Could you check a few things on this drawing? It's one solid part, dimensions in mm from its lowest x, y, z. A direction names the side the tool comes from. Round coordinates to 2 decimals unless told otherwise and drop trailing zeros. Loops run counter-clockwise (first coordinate to the right, second up) from the corner with the lowest first, then second, coordinate; pieces in that order, holes last. Notation, with made-up numbers: (47.5, 34) -> (82.5, 34) arc R27 cw to (82.5, 62) -> close; hole circle Ø5 at (63, 83). An arc over 180 degrees is marked (long way). Use one line per item in the form item = value. Start each with the question number.
Item 1: If we section it at D-D (x = 22): Write out the boundary of the cut face in (y, z), then the cut area to 3 significant figures.
Item 2: If we section it at A-A (x = 4): Write out the boundary of the cut face in (y, z).
Item 3: If we section it at B-B (z = 6.75): Write out the boundary of the cut face in (x, y), then the cut area to 3 significant figures.
Item 4: If I drill on L1, parallel to X at y = 6.75, z = 8; L2, parallel to Y at x = 4, z = 1.3; L3, parallel to Y at x = 30, z = 1.3, over which ranges is the centre line in solid material (lowest first)? Write a range as [from, to].
Item 5: For the marked faces 1, 2, 3, 4 and 5, which set-ups out of +Z, -Z, +X, -X, +Y, -Y let a thin tool reach every point of the face, with its end or its side?
Item 6: Thinking about a two-plate mould opening in X: for the marked faces 6, 7, 8 and 9, which applies, released by +X, released by -X, zero draft, split by the parting line, or undercut?
Item 7: If we section it at C-C (y = 17): Write out the boundary of the cut face in (x, z).
Item 8: I'm going to push flat-ended pins straight in: pin 1 Ø4.5 at (y, z) = (5, 6.5) entering from +X; pin 2 Ø1.2 at (x, y) = (15.5, 6) entering from +Z; pin 3 Ø3 at (x, z) = (12.5, 5.5) entering from -Y; pin 4 Ø5 at (y, z) = (11, 9) entering from -X. Where does each tip first touch, or does it pass through?
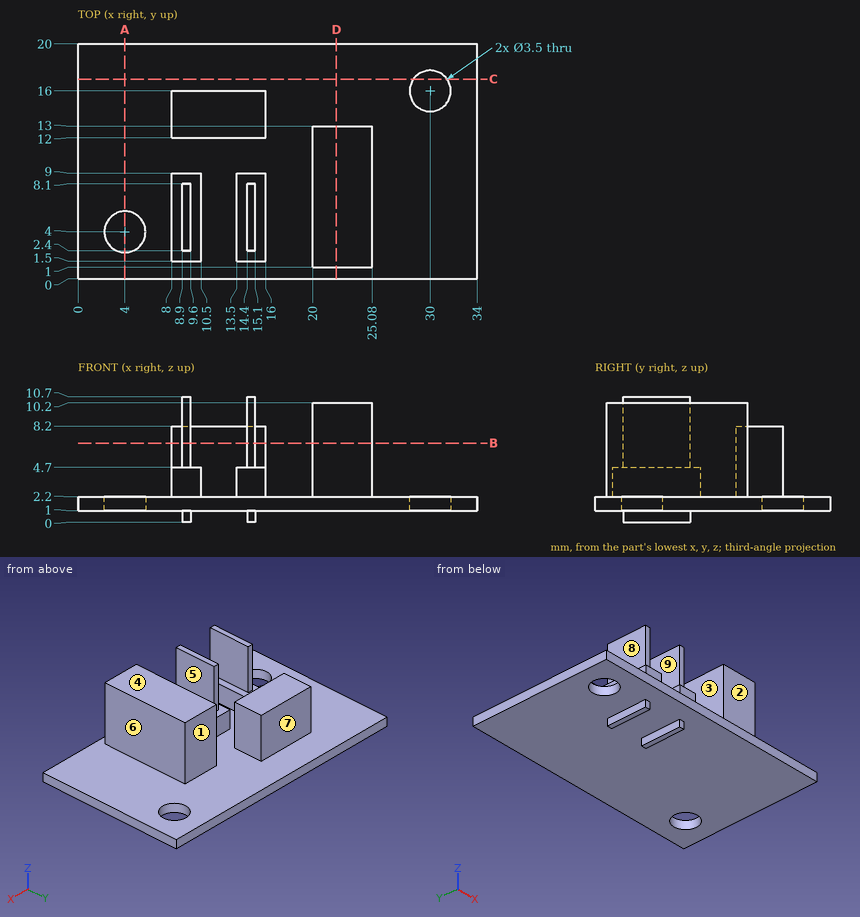
Values found:
q1.outline = (0, 1) -> (20, 1) -> (20, 2.2) -> (13, 2.2) -> (13, 10.2) -> (1, 10.2) -> (1, 2.2) -> (0, 2.2) -> close
q1.area = 120 mm2
q2.outline = (0, 1) -> (2.25, 1) -> (2.25, 2.2) -> (0, 2.2) -> close; (5.75, 1) -> (20, 1) -> (20, 2.2) -> (5.75, 2.2) -> close
q3.outline = (8, 12) -> (16, 12) -> (16, 16) -> (8, 16) -> close; (8.9, 2.4) -> (9.6, 2.4) -> (9.6, 8.1) -> (8.9, 8.1) -> close; (14.4, 2.4) -> (15.1, 2.4) -> (15.1, 8.1) -> (14.4, 8.1) -> close; (20, 1) -> (25.08, 1) -> (25.08, 13) -> (20, 13) -> close
q3.area = 101 mm2
q4.L1 = [8.9, 9.6], [14.4, 15.1], [20, 25.08]
q4.L2 = [0, 2.25], [5.75, 20]
q4.L3 = [0, 14.25], [17.75, 20]
q5.face_1 = +Z, +X, +Y
q5.face_2 = +Z, +X, -X, -Y
q5.face_3 = +Z, +Y, -Y
q5.face_4 = +Z, +X, +Y, -Y
q5.face_5 = +Z, -Y
q6.face_6 = released by +X
q6.face_7 = zero draft
q6.face_8 = released by -X
q6.face_9 = undercut
q7.outline = (0, 1) -> (28.56, 1) -> (28.56, 2.2) -> (0, 2.2) -> close; (31.44, 1) -> (34, 1) -> (34, 2.2) -> (31.44, 2.2) -> close
q8.pin_1 = 25.08
q8.pin_2 = 10.7
q8.pin_3 = 1.5
q8.pin_4 = 8
